```python
from build123d import *

# Parameters (mm, degrees)
BOSS_EXTRUDE1_DEPTH = 7
BOSS_EXTRUDE3_DEPTH = 15


with BuildPart() as part:
    # Sketch2 → Boss-Extrude1 (new body)
    with BuildSketch(Plane.XY):
        with BuildLine():
            Line((46.285916799, 119.634724339), (134.396340404, 139.050413551))
            Line((134.396340404, 139.050413551), (134.39379389, 182.38704377))
            Line((134.39379389, 182.38704377), (120.894388682, 182.386250529))
            Line((120.894388682, 182.386250529), (120.894655408, 177.847108131))
            Line((120.894655408, 177.847108131), (120.895456025, 177.847108131))
            Line((120.895456025, 177.847108131), (120.895456025, 154.100245399))
            ThreePointArc((120.895456025, 154.100245399), (115.895456025, 149.100245399), (110.895456025, 154.100245399))
            Line((110.895456025, 154.100245399), (110.895456025, 164.221886849))
            Line((110.895456025, 164.221886849), (110.894388699, 182.385662916))
            Line((110.894388699, 182.385662916), (98.145136748, 182.384913754))
            Line((98.145136748, 182.384913754), (78.980988049, 187.822713754))
            Line((78.980988049, 187.822713754), (78.151086328, 185.147461295))
            Line((78.151086328, 185.147461295), (88.076413708, 182.068482243))
            add(Edge.make_bspline(
                [(83.678693998, 168.728153838), (88.77463375, 174.312097996), (88.076413708, 182.068482243)],
                knots=[0, 0, 0, 1, 1, 1], degree=2))
            Line((83.678693998, 168.728153838), (73.917241092, 171.824383576))
            Line((73.917241092, 171.824383576), (73.018341013, 168.990430176))
            Line((73.018341013, 168.990430176), (77.298136398, 167.632924294))
            Line((77.298136398, 167.632924294), (83.134894854, 162.46237946))
            Line((83.134894854, 162.46237946), (84.589439396, 156.392019708))
            Line((84.589439396, 156.392019708), (46.285916799, 143.661523495))
            Line((46.285916799, 143.661523495), (46.285916799, 119.634724339))
        make_face()
    extrude(amount=BOSS_EXTRUDE1_DEPTH)

    # Sketch2<5> → Boss-Extrude3 (add)
    with BuildSketch(Plane.XY):
        Polygon((87.058472282, 182.384262288), (88.076413708, 182.068482243), (99.075977115, 178.656259752), (110.895456025, 164.221886849), (110.895184282, 168.846419808), (110.894388699, 182.385662916), (98.145136748, 182.384913754), align=None)
        Polygon((78.151086328, 185.147461295), (87.058472282, 182.384262288), (98.145136748, 182.384913754), (78.980988049, 187.822713754), align=None)
        with BuildLine():
            Line((46.285916799, 143.661523495), (46.285916799, 140.73837931))
            Line((46.285916799, 140.73837931), (83.134894854, 152.985445474))
            add(Edge.make_bspline(
                [(83.134894854, 152.985445474), (84.174927516, 153.23074968), (85.840748742, 154.28331709), (87.795600381, 156.094817729), (88.836774052, 158.514861149), (89.609824294, 162.728645553), (87.029154532, 166.875865112), (84.288075, 168.507673549), (83.678693998, 168.728153838)],
                knots=[0, 0, 0, 0, 0.137401343, 0.255123746, 0.340171857, 0.476918897, 0.801613812, 0.887468334, 0.887468334, 0.887468334, 0.887468334], degree=3))
            Line((83.678693998, 168.728153838), (83.308823, 168.845473012))
            add(Edge.make_bspline(
                [(83.308823, 168.845473012), (82.615828523, 169.034245679), (81.877979683, 169.060179847), (81.093974035, 168.846419773)],
                knots=[0.904634429, 0.904634429, 0.904634429, 0.904634429, 1, 1, 1, 1], degree=3))
            Line((81.093974035, 168.846419773), (77.298136398, 167.632924294))
            Line((77.298136398, 167.632924294), (83.134894854, 162.46237946))
            Line((83.134894854, 162.46237946), (84.589439396, 156.392019708))
            Line((84.589439396, 156.392019708), (46.285916799, 143.661523495))
        make_face()
        with BuildLine():
            Line((73.018341013, 168.990430176), (77.298136398, 167.632924294))
            Line((77.298136398, 167.632924294), (81.093974035, 168.846419773))
            add(Edge.make_bspline(
                [(83.308823, 168.845473012), (82.615828523, 169.034245679), (81.877979683, 169.060179847), (81.093974035, 168.846419773)],
                knots=[0.904634429, 0.904634429, 0.904634429, 0.904634429, 1, 1, 1, 1], degree=3))
            Line((83.308823, 168.845473012), (73.917241092, 171.824383576))
            Line((73.917241092, 171.824383576), (73.018341013, 168.990430176))
        make_face()
        with BuildLine():
            Line((119.308499738, 139.814661997), (46.285916799, 123.723673918))
            Line((46.285916799, 123.723673918), (46.285916799, 119.634724339))
            Line((46.285916799, 119.634724339), (134.396340404, 139.050413551))
            Line((134.396340404, 139.050413551), (134.394880743, 163.890947893))
            Line((134.394880743, 163.890947893), (134.0570987, 163.890947893))
            add(Edge.make_bspline(
                [(133.108709045, 162.9170571), (133.328673606, 163.695225929), (134.0570987, 163.890947893)],
                knots=[0, 0, 0, 1, 1, 1], degree=2))
            add(Edge.make_bspline(
                [(119.308499738, 139.814661997), (123.463953154, 140.563007639), (134.082921071, 146.527888), (130.556655112, 158.461365551), (133.108709045, 162.9170571)],
                knots=[0, 0, 0, 0, 0.463455576, 1, 1, 1, 1], degree=3))
        make_face()
    extrude(amount=BOSS_EXTRUDE3_DEPTH)


solid = part.part
```
Work out the finished part from the listing and answer in its coordinate system (mm). A direction names the side the tool comes from. Give positions to 0.01 mm unless a question says otherwise; leave off trailing zeros. Loops run counter-clockwise (first coordinate to the right, second up) from the corner with the lowest first, then second, coordinate; pieces in that order, holes last. Notation, with made-up numbers: (-39.5, -8) -> (1.5, -8) arc R14 ccw to (1.5, 3) -> close; hole circle Ø7 at (67, -12.5). An arc over 180 degrees is marked (long way). Use CSV: the item, a comma, the result in double quotes.
1. The part is cut by section B-B (z = 11.5). State how many separate pieces and enclosed holes the cut face has, then the cut area to 3 significant figures.
Found:
separate pieces,"3"
enclosed holes,"0"
area,"846 mm^2"
2. The mould has two halves that part along Y. Classify faces 1 (the flat face through (80.18, 165.08, 7.4)), 2 (the flat face through (73.474, 170.427, 7.395)), 3 (the flat face through (120.895, 166, 3)): +Y half, -Y half, draft (parallel to the pull), parting line (faces both ways), or undercut.
Found:
face 1,"undercut"
face 2,"+Y half"
face 3,"draft"
3. Straight lines are drawn through the part: line 1 (Y direction, x = 74, z = 9); line 2 (Y direction, x = 80.5, z = 1); line 3 (Y direction, x = 104.5, z = 12). For each, find the intervals that lie inside material, in ascending order.
Found:
line 1,"125.74 to 129.83, 149.95 to 152.87, 168.68 to 171.8"
line 2,"127.17 to 155.03, 164.8 to 169.74, 184.42 to 187.39"
line 3,"132.46 to 136.55, 172.03 to 182.39"
4. The part is cut by section D-D (x = 108). Write down the section's boundary in (y, z), then the cut area to 3 significant figures.
Found:
outline,"(133.23, 0) -> (182.39, 0) -> (182.39, 15) -> (167.76, 15) -> (167.76, 7) -> (137.32, 7) -> (137.32, 15) -> (133.23, 15) -> close"
area,"494 mm^2"
5. A tool of negligible diameter and unlimited length cuts with its end or side. For faces 4 (the flat face through (83.85, 159.47, 7.4)), 5 (the flat face through (83.308, 131.882, 10.944)), 6 (the flat face through (104.903, 171.54, 10.944)), from which of +Z, -Z, +X, -X, +Y, -Y can it reach the whole face along a straight path? Write none if from no direction.
Found:
face 4,"+Z, -Z, -X"
face 5,"+Z, -X"
face 6,"+Z"
6. The part is cut by section C-C (y = 126). Write down the section's boundary in (x, z), then the cut area to 3 significant figures.
Found:
outline,"(46.29, 0) -> (75.17, 0) -> (75.17, 15) -> (56.62, 15) -> (56.62, 7) -> (46.29, 7) -> close"
area,"351 mm^2"
7. The part is cut by section A-A (x = 55). Write down the section's boundary in (y, z).
Found:
outline,"(121.55, 0) -> (146.56, 0) -> (146.56, 15) -> (143.63, 15) -> (143.63, 7) -> (125.64, 7) -> (125.64, 15) -> (121.55, 15) -> close"
8. Flat-ended cylindrical pins translate along their axes: pin 1 Ø2.5 at (y, z) = (175.5, 11.5) entering from +X; pin 2 Ø6 at (x, y) = (95.5, 164) entering from -Z; pin 3 Ø2 at (x, z) = (102, 2) entering from -Y; pin 4 Ø4 at (x, z) = (106, 4.5) entering from +Y. Find the tip coordinate at first contact, or state that the pin passes through.
Found:
pin 1,"x = 110.89"
pin 2,"z = 0"
pin 3,"y = 131.69"
pin 4,"y = 182.39"
